Check sheet for the drawn part. Datum: minimum x, y, z corner. Units: mm. A direction names the side the tool comes from. Round coordinates to 2 decimals unless told otherwise and drop trailing zeros. Write each loop counter-clockwise with the first axis right and the second up, starting at its lowest first coordinate (ties: lowest second). Pieces come first, ordered by that corner, then holes. Notation, with made-up numbers: (13.5, 29.5) - (63.5, 29.5) arc R35 cw to (63.5, 63.5) - close; hole circle Ø7 at (-39, 47). An arc over 180 degrees is marked (long way). Answer as a JSON object with one key per item and string values.
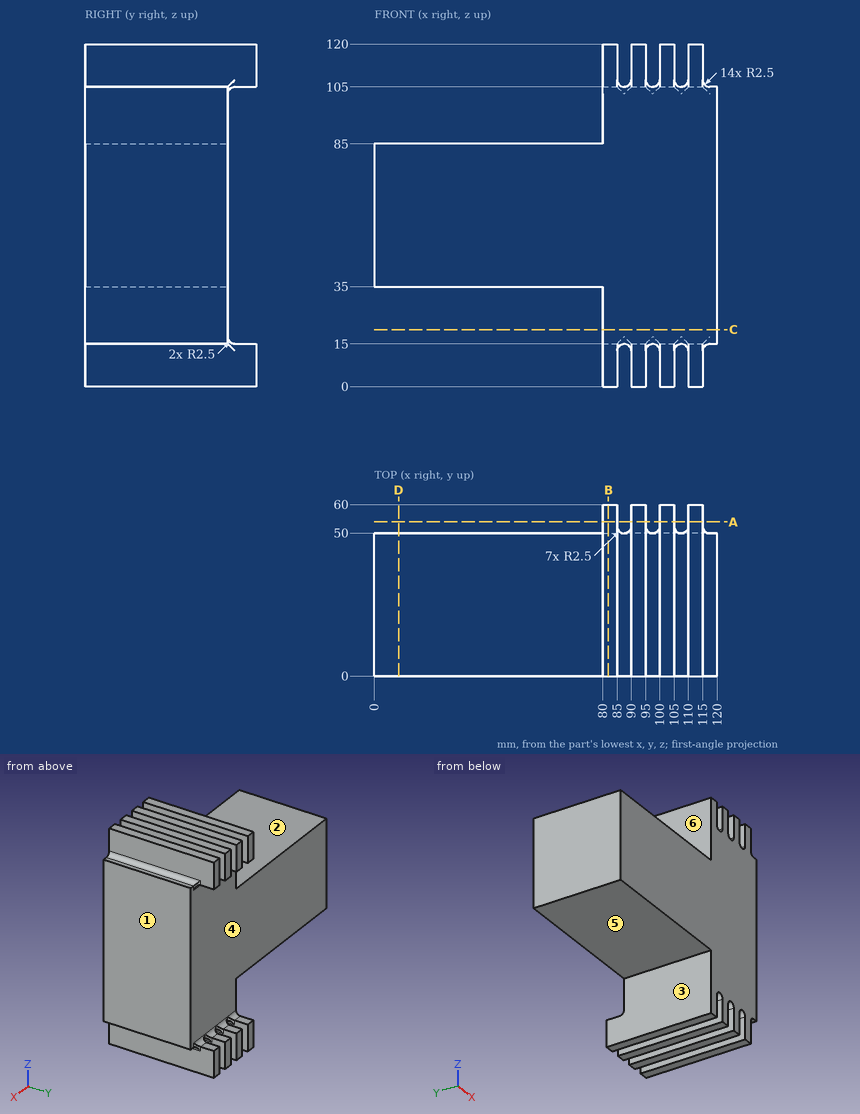
1. Go/stop test with flat-tipped pins: pin 1 (4.5 mm diameter, centred on y = 34, z = 6.5, fed in from -X); pin 2 (2 mm diameter, centred on x = 118.5, y = 15, fed in from -Z); pin 3 (12 mm diameter, centred on y = 15.5, z = 112, fed in from +X). Record where each tip stops, or that it passes through.
Completed:
{"pin 1": "stops at x = 80", "pin 2": "stops at z = 15", "pin 3": "stops at x = 115.5"}
2. Cross-section at C-C (z = 20). Record the boundary of the cut face in (x, y).
Completed:
{"outline": "(80, 0) - (120, 0) - (120, 50) - (80, 50) - close"}
3. Access from +Z, -Z, +X, -X, +Y, -Y to the whole of each face (thin tool, end or side, straight path). Record for the marked faces 1, 2 and 3.
Completed:
{"face 1": "+Z, -Z, +X, +Y, -Y", "face 2": "+Z, -X, +Y, -Y", "face 3": "-Z, -X, +Y, -Y"}
4. Cross-section at B-B (x = 82). Record the boundary of the cut face in (y, z), plus the area to 3 significant figures.
Completed:
{"outline": "(0, 0) - (60, 0) - (60, 15) - (52.5, 15) arc R2.5 cw to (50, 17.5) - (50, 102.5) arc R2.5 cw to (52.5, 105) - (60, 105) - (60, 120) - (0, 120) - close", "area": "6,300 mm^2"}
5. Cross-section at A-A (y = 54). Count the separate pieces of the cut face and the enclosed holes in it, plus the area to 3 significant figures.
Completed:
{"separate pieces": "8", "enclosed holes": "0", "area": "600 mm^2"}
6. Mould release check, pull along Z, two halves, no side actions. Record for the marked faces 4, 5 and 6: released by +Z, released by -Z, zero draft, split by the parting line, or undercut.
Completed:
{"face 4": "undercut", "face 5": "released by -Z", "face 6": "zero draft"}
7. Material ranges on probe 1 along X at (y, z) = (18.5, 11.5); probe 2 along X at (y, z) = (18, 13.5); probe 3 along X at (y, z) = (39.5, 86.5), recorded low to high. Write a range as from..to.
Completed:
{"probe 1": "x = 80..85, 90..95, 100..105, 110..115", "probe 2": "x = 80..85.21, 89.79..95.21, 99.79..105.21, 109.79..115.21", "probe 3": "x = 80..120"}
8. Cross-section at D-D (x = 8.5). Record the boundary of the cut face in (y, z), plus the area to 3 significant figures.
Completed:
{"outline": "(0, 35) - (50, 35) - (50, 85) - (0, 85) - close", "area": "2,500 mm^2"}
